from build123d import *

# Parameters (mm, degrees)
CROQUIS1_W                                   = 205
CROQUIS1_H                                   = 155
SALIENTE_EXTRUIR1_DEPTH                      = 5
REDONDEO1_DEPTH                              = 205
REDONDEO1_START                              = -156
REDONDEO1_2_DEPTH                            = 157
CROQUIS2_R                                   = 1.5
CORTAR_EXTRUIR1_DEPTH                        = 3
PERFORADOR_PARA_ROSCAR_HELICOIL_DE_M41_D     = 4.2
PERFORADOR_PARA_ROSCAR_HELICOIL_DE_M41_DEPTH = 3.25
PERFORADOR_PARA_ROSCAR_HELICOIL_DE_M41_TIP   = 1.2618073


with BuildPart() as part:
    # Croquis1 → Saliente-Extruir1 (new body)
    with BuildSketch(Plane(origin=(0, 0, 0), x_dir=(1, 0, 0), z_dir=(0, 1, 0))):
        with Locations((102.5, 77.5)):
            Rectangle(CROQUIS1_W, CROQUIS1_H)
    extrude(amount=SALIENTE_EXTRUIR1_DEPTH)

    # Redondeo1: read off the stored shape, not the designer's step
    # Redondeo1 outline → Redondeo1 (cut)
    with BuildSketch(Plane.YZ):
        with BuildLine():
            Line((5, -155), (5, -152.5))
            add(Edge.make_bspline(
                [(5, -152.5), (5, -155), (2.5, -155)],
                knots=[0, 0, 0, 1, 1, 1], degree=2, weights=[1, 0.353553391, 1]))
            Line((2.5, -155), (5, -155))
        make_face()
        with BuildLine():
            add(Edge.make_bspline(
                [(5, -2.5), (5, 0), (2.5, 0)],
                knots=[0, 0, 0, 1, 1, 1], degree=2, weights=[1, 0.353553391, 1]))
            Line((5, -2.5), (5, 0))
            Line((5, 0), (2.5, 0))
        make_face()
    extrude(amount=REDONDEO1_DEPTH, mode=Mode.SUBTRACT)

    # Redondeo1 2 outline → Redondeo1 2 (cut)
    with BuildSketch(Plane.XY.offset(REDONDEO1_START)):
        with BuildLine():
            Line((205, 5), (202.5, 5))
            add(Edge.make_bspline(
                [(202.5, 5), (205, 5), (205, 2.5)],
                knots=[0, 0, 0, 1, 1, 1], degree=2, weights=[1, 0.353553391, 1]))
            Line((205, 2.5), (205, 5))
        make_face()
        with BuildLine():
            add(Edge.make_bspline(
                [(2.5, 5), (0, 5), (0, 2.5)],
                knots=[0, 0, 0, 1, 1, 1], degree=2, weights=[1, 0.353553391, 1]))
            Line((2.5, 5), (0, 5))
            Line((0, 5), (0, 2.5))
        make_face()
    extrude(amount=REDONDEO1_2_DEPTH, mode=Mode.SUBTRACT)

    # Croquis2 → Cortar-Extruir1 (cut)
    with BuildSketch(Plane(origin=(0, 5, 0), x_dir=(1, 0, 0), z_dir=(0, 1, 0))):
        with Locations(Location((77.5, 77.5, 0), (0, 0, 270))):
            Circle(CROQUIS2_R)
        with Locations(Location((102.5, 102.5, 0), (0, 0, 270))):
            Circle(CROQUIS2_R)
        with Locations(Location((127.5, 77.5, 0), (0, 0, 270))):
            Circle(CROQUIS2_R)
        with Locations(Location((102.5, 52.5, 0), (0, 0, 270))):
            Circle(CROQUIS2_R)
    extrude(amount=-CORTAR_EXTRUIR1_DEPTH, mode=Mode.SUBTRACT)

    # Perforador para roscar Helicoil de M41
    with Locations(Plane(origin=(0, 5, 0), x_dir=(1, 0, 0), z_dir=(0, 1, 0))):
        with Locations((77.5, 77.5), (102.5, 102.5), (127.5, 77.5), (102.5, 52.5)):
            Hole(PERFORADOR_PARA_ROSCAR_HELICOIL_DE_M41_D / 2, depth=PERFORADOR_PARA_ROSCAR_HELICOIL_DE_M41_DEPTH)
            with Locations((0, 0, -(PERFORADOR_PARA_ROSCAR_HELICOIL_DE_M41_DEPTH + PERFORADOR_PARA_ROSCAR_HELICOIL_DE_M41_TIP / 2))):  # 118° drill point
                Cone(0, PERFORADOR_PARA_ROSCAR_HELICOIL_DE_M41_D / 2, PERFORADOR_PARA_ROSCAR_HELICOIL_DE_M41_TIP, mode=Mode.SUBTRACT)


solid = part.part
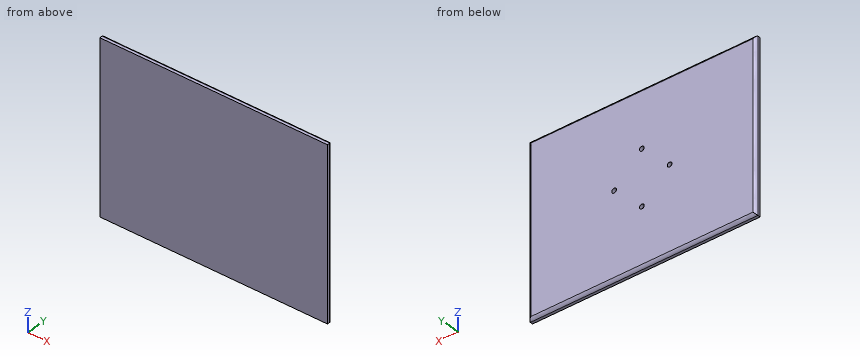
Work out the finished part from the listing and answer in its coordinate system (mm). Round coordinates to 2 decimals unless told otherwise and drop trailing zeros. Write each question's results on one line, items separated by ' | '.
Item 1: Find the intervals of material crossed by line 1 along Z through (x, y) = (102.5, 2.5); line 2 along Z through (x, y) = (102.5, 4.05); line 3 along Z through (x, y) = (127.5, 2.7), in increasing order. Write a range as [from, to].
Result set:
line 1: [-155, -104.6], [-100.4, -54.6], [-50.4, 0] | line 2: [-154.1, -104.6], [-100.4, -54.6], [-50.4, -0.9] | line 3: [-154.97, -79.6], [-75.4, -0.03]
Item 2: A cutting plane is placed at A-A, the plane y = 4.15. Count the separate pieces of the cut face and the enclosed holes in it, plus the area to 3 significant figures.
Result set:
separate pieces: 1 | enclosed holes: 4 | area: 31,000 mm^2
Item 3: Flat-ended cylindrical pins translate along their axes: P1, Ø3.5, axis at x = 127.5, z = -77.5, coming from the +Y side; P2, Ø2.5, axis at x = 77.5, z = -77.5, coming from the +Y side. Find the tip coordinate at first contact, or state that the pin passes through.
Result set:
P1: y = 1.54 | P2: y = 1.24
